from build123d import *

# Parameters (mm, degrees)
BOSS_EXTRUDE1_DEPTH = 1.6
DRAFT1_ANGLE        = 9.10617604
SKETCH2_W           = 3.45
SKETCH2_H           = 1.4
HOLE1_D             = 4.2
HOLE1_DEPTH         = 3
FILLET1_R           = 1.5


with BuildPart() as part:
    # Sketch1 → Boss-Extrude1 (new body)
    with BuildSketch(Plane.XY.offset(1.6)):
        Polygon((3, -5), (6.092206474, -4.504366896), (7.5, 4.278719262), (3, 5), (-3, 5), (-7.5, 4.278719262), (-7.5, -4.278719262), (-3, -5), align=None)
    extrude(amount=-BOSS_EXTRUDE1_DEPTH)

    # Draft1
    draft1_faces = [part.faces().sort_by_distance(p)[0] for p in [
        (6.796103237, -0.112823817, 0.8),
    ]]
    draft(draft1_faces, Plane(origin=(7.5, 4.278719262, 0), x_dir=(0.987396753, -0.158264502, 0), z_dir=(0.158264502, 0.987396753, 0)), DRAFT1_ANGLE)

    # Sketch2 → Revolve1 (revolve)
    with BuildSketch(Plane.XZ):
        with Locations((1.725, 2.3)):
            Rectangle(SKETCH2_W, SKETCH2_H)
    revolve(axis=Axis((0, 0, 3), (0, 0, -1)))

    # Hole1
    with Locations(Plane.XY.offset(3)):
        with Locations((0, 0)):
            Hole(HOLE1_D / 2, depth=HOLE1_DEPTH)

    # Fillet1
    fillet1_edges = [part.edges().sort_by_distance(p)[0] for p in [
        (-7.5, -4.278719262, 0.8),
        (-7.5, 4.278719262, 0.8),
        (7.5, 4.278719262, 0.8),
        (7.5, -4.278719262, 0.8),
    ]]
    fillet(fillet1_edges, radius=FILLET1_R)


solid = part.part
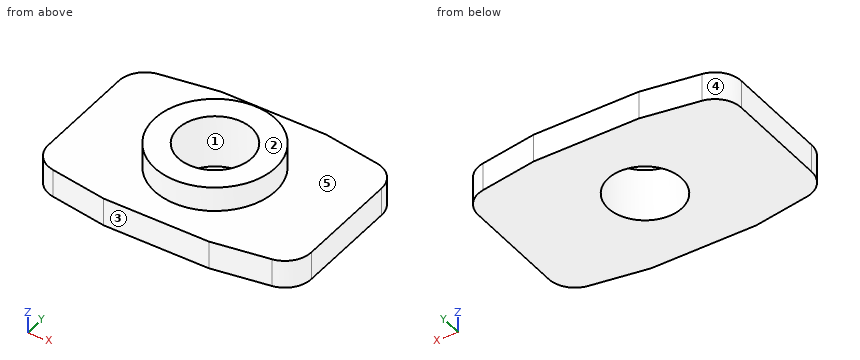
The listing builds one solid part. Answer for the finished solid, in the listing's coordinates (mm). Face numbers are marked on the shaded views. A direction names the side the tool comes from. Coordinates: 2 decimals unless noted, no trailing zeros. Order: outer loops, then holes, each group sorted by start corner. A loop starts at its lowest first (then second) coordinate and runs counter-clockwise, first axis right, second up.
Q1. A cutting plane is placed at C-C, the plane z = 0.7. Write down the section's boundary in (x, y), and give its area (3 significant figures).
Q2. For a pull along Y with two mould halves and no side action, classify the marked faces 1, 2 and 3 as pulls with the +Y half, pulls with the -Y half, needs draft (parallel to the pull), parting line crosses it, or undercut.
Q3. A cutting plane is placed at D-D, the plane x = 5.75. Write down the section's boundary in (y, z), and give its area (3 significant figures).
Q4. Which of the six approach directions +Z, -Z, +X, -X, +Y, -Y give full straight-line access (tool end or side, diameter ignored) to the marked faces 4 and 5?
Q5. A cutting plane is placed at B-B, the plane y = 0. Write down the section's boundary in (x, z), and give its area (3 significant figures).
Q6. Consider line 1 (Y direction, x = 0, z = 1.95); line 2 (Y direction, x = 0, z = 0.85); line 3 (Z direction, x = 6.75, y = -0.5). Determine where each line is inside the solid, lowest interval first.
Q7. A cutting plane is placed at A-A, the plane x = 0. Write down the section's boundary in (y, z).
Q8. Given P1, Ø5, axis at x = 0, y = 0, coming from the +Z side, flat-ended and moving along its own axis, determine where the tip first touches the part or whether it passes through.
Answers follow:
1. outline: (-7.5, -3) arc R1.5 ccw to (-6.24, -4.48) - (-3, -5) - (3, -5) - (6.24, -4.48) arc R1.5 ccw to (7.5, -3) - (7.5, 3) arc R1.5 ccw to (6.24, 4.48) - (3, 5) - (-3, 5) - (-6.24, 4.48) arc R1.5 ccw to (-7.5, 3) - close; hole circle Ø4.2 at (0, 0)
1. area: 128 mm2
2. face 1: undercut
2. face 2: needs draft
2. face 3: pulls with the -Y half
3. outline: (-4.56, 0) - (4.56, 0) - (4.56, 1.6) - (-4.56, 1.6) - close
3. area: 14.6 mm2
4. face 4: +Z, -Z, -X, +Y
4. face 5: +Z
5. outline: (-7.5, 0) - (-2.1, 0) - (-2.1, 3) - (-3.45, 3) - (-3.45, 1.6) - (-7.5, 1.6) - close; (2.1, 0) - (7.5, 0) - (7.5, 1.6) - (3.45, 1.6) - (3.45, 3) - (2.1, 3) - close
5. area: 21.1 mm2
6. line 1: y = -3.45 to -2.1, 2.1 to 3.45
6. line 2: y = -5 to -2.1, 2.1 to 5
6. line 3: z = 0 to 1.6
7. outline: (-5, 0) - (-2.1, 0) - (-2.1, 3) - (-3.45, 3) - (-3.45, 1.6) - (-5, 1.6) - close; (2.1, 0) - (5, 0) - (5, 1.6) - (3.45, 1.6) - (3.45, 3) - (2.1, 3) - close
8. P1: stops at z = 3
